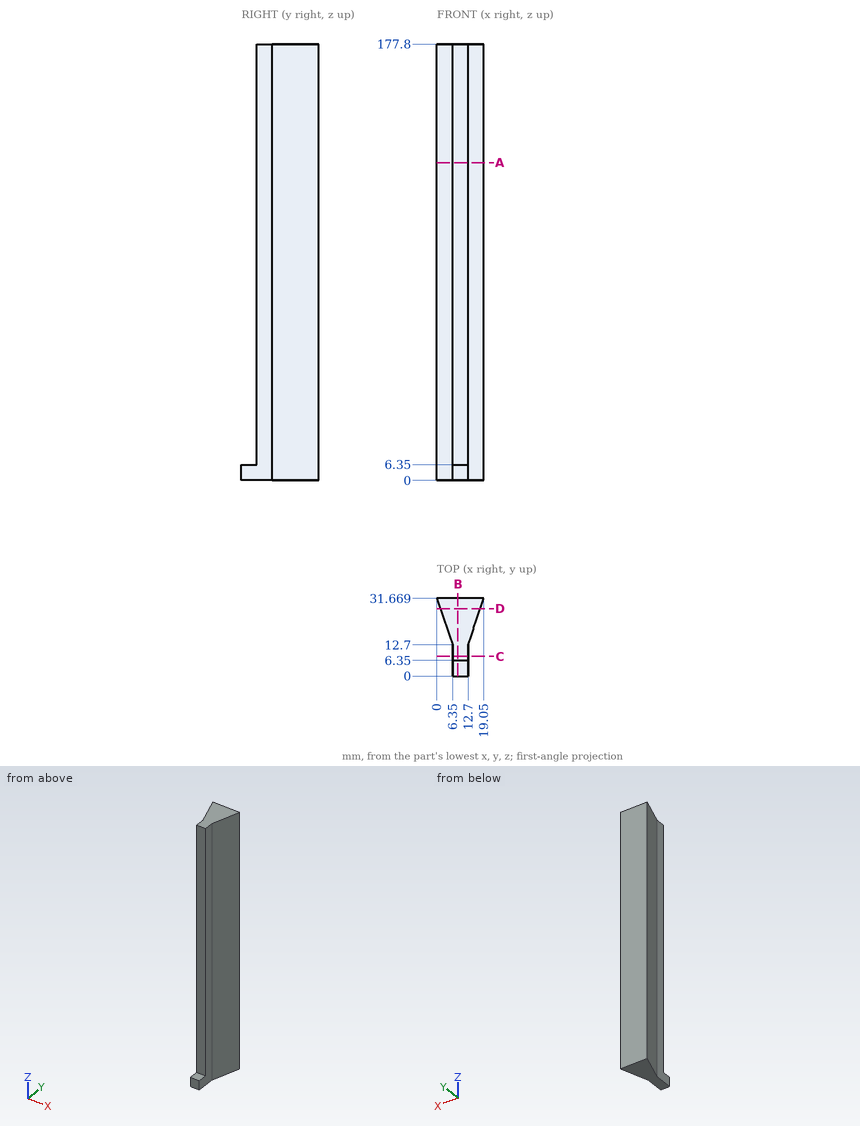
Input: dimensioned drawing with shaded views. Units: mm. Origin: part minimum x, y, z. Coordinates: 2 decimals unless noted, no trailing zeros. Loops run counter-clockwise (first coordinate to the right, second up) from the corner with the lowest first, then second, coordinate; pieces in that order, holes last. Notation, with made-up numbers: M 39,16 L 56,16 A30 ccw 56,42 Z; hole C 4,-21.75 d4. An arc over 180 degrees is marked long. Use a Markdown table: item, result. Add a question column.
1) Section A-A, the plane z = 129.5. Return the cut outline in (x, y), plus the area to 3 significant figures.
2) Pin query (flat end, axial travel): P1, Ø1.5, axis at y = 8.5, z = 130.5, coming from the -X side; P2, Ø6, axis at x = 10.5, z = 70.5, coming from the -Y side; P3, Ø3, axis at x = 8.5, z = 110, coming from the -Y side. Return the tip coordinate at first contact, or that it passes through.
3) Section B-B, the plane x = 8.5. Return the cut outline in (y, z), plus the area to 3 significant figures.
4) Line query: L1, parallel to X at y = 6.5, z = 44; L2, parallel to Y at x = 7.5, z = 59; L3, parallel to Z at x = 9, y = 2. Output: solid intervals per line, ascending. Write a range as from..to.
5) Section C-C, the plane y = 8. Return the cut outline in (x, z).
6) Section D-D, the plane y = 27.5. Return the cut outline in (x, z) (1 decimal).
Answer below:
| question | item | result |
|---|---|---|
| 1 | outline | M 0,31.67 L 6.35,12.7 L 6.35,6.35 L 12.7,6.35 L 12.7,12.7 L 19.05,31.67 Z |
| 1 | area | 281 mm2 |
| 2 | P1 | x = 6.35 |
| 2 | P2 | y = 6.35 |
| 2 | P3 | y = 6.35 |
| 3 | outline | M 0,0 L 31.67,0 L 31.67,177.8 L 6.35,177.8 L 6.35,6.35 L 0,6.35 Z |
| 3 | area | 4,540 mm2 |
| 4 | L1 | 6.35..12.7 |
| 4 | L2 | 6.35..31.67 |
| 4 | L3 | 0..6.35 |
| 5 | outline | M 6.35,0 L 12.7,0 L 12.7,177.8 L 6.35,177.8 Z |
| 6 | outline | M 1.4,0 L 17.7,0 L 17.7,177.8 L 1.4,177.8 Z |
